```python
from build123d import *

# Parameters (mm, degrees)
SKETCH1_R           = 10.31875
BOSS_EXTRUDE1_DEPTH = 9.525
SKETCH2_R           = 18.2626
BOSS_EXTRUDE2_DEPTH = 19.05
CUT_EXTRUDE1_START  = -2.38125
SKETCH3_OUTSIDE_W   = 50.332
SKETCH3_OUTSIDE_H   = 50.332
SKETCH3_OUTSIDE_R   = 15.1638
CUT_EXTRUDE1_DEPTH  = 14.2875
SKETCH4_R           = 4.7625
CUT_EXTRUDE2_DEPTH  = 14.2875
CIRPATTERN1_COUNT   = 10
CUT_EXTRUDE3_DEPTH  = 39.517213587


with BuildPart() as part:
    # Sketch1 → Boss-Extrude1 (new body)
    with BuildSketch(Plane(origin=(0, 0, 0), x_dir=(0, 0, -1), z_dir=(1, 0, 0))):
        with Locations(Location((0, 0, 0), (0, 0, 180))):
            Circle(SKETCH1_R)
    extrude(amount=BOSS_EXTRUDE1_DEPTH)

    # Sketch2 → Boss-Extrude2 (add)
    with BuildSketch(Plane(origin=(9.525, 0, 0), x_dir=(0, 0, -1), z_dir=(1, 0, 0))):
        with Locations(Location((0, 0, 0), (0, 0, 180))):
            Circle(SKETCH2_R)
    extrude(amount=BOSS_EXTRUDE2_DEPTH)

    # Sketch3 outside → Cut-Extrude1 (cut)
    with BuildSketch(Plane(origin=(28.575, 0, 0), x_dir=(0, 0, -1), z_dir=(1, 0, 0)).offset(CUT_EXTRUDE1_START)):
        Rectangle(SKETCH3_OUTSIDE_W, SKETCH3_OUTSIDE_H)
        Circle(SKETCH3_OUTSIDE_R, mode=Mode.SUBTRACT)
    extrude(amount=-CUT_EXTRUDE1_DEPTH, mode=Mode.SUBTRACT)

    # Sketch4 → Cut-Extrude2 (cut)
    with BuildSketch(Plane.ZY.offset(-26.19375)):
        with Locations((-12.712096792, 8.267008262)):
            Circle(SKETCH4_R)
    cut_extrude2 = extrude(amount=CUT_EXTRUDE2_DEPTH, mode=Mode.SUBTRACT)

    # CirPattern1: Cut-Extrude2 ×10 about axis
    cirpattern1_axis = Axis((0, 0, 0), (1, 0, 0))
    for i in range(1, CIRPATTERN1_COUNT):
        add(cut_extrude2.rotate(cirpattern1_axis, i * 360 / CIRPATTERN1_COUNT), mode=Mode.SUBTRACT)

    # Sketch5 → Cut-Extrude3 (cut, through all)
    with BuildSketch(Plane.ZY):
        Polygon((-7.332348419, 0), (-3.666174209, -6.35), (3.666174209, -6.35), (7.332348419, 0), (3.666174209, 6.35), (-3.666174209, 6.35), align=None)
    extrude(amount=-CUT_EXTRUDE3_DEPTH, mode=Mode.SUBTRACT)


solid = part.part
```
Can you work these out from the model? Positions are in its coordinate system, mm. A direction names the side the tool comes from. Round coordinates to 2 decimals unless told otherwise and drop trailing zeros. Order: outer loops, then holes, each group sorted by start corner. A loop starts at its lowest first (then second) coordinate and runs counter-clockwise, first axis right, second up. Notation, with made-up numbers: (21.5, 70) -> (35.5, 70) arc R9 ccw to (35.5, 74) -> close; hole circle Ø6 at (26, 68.25). An arc over 180 degrees is marked (long way). Return JSON: item names as keys, results as strings. Group by question number.
1. If we section it at B-B, the plane z = 0: Write out the boundary of the cut face in (x, y) (3 decimals), then the cut area to 3 significant figures.
2. I need wall thicknesses on line 1 (X direction, y = 7.5, z = 12) (3 decimals); line 2 (Y direction, x = 2.5, z = 3); line 3 (Y direction, x = 5.5, z = 0). Which ranges of each line are inside material? Lowest first, please. Write a range as [from, to].
3. Which directions (+Z, -Z, +X, -X, +Y, -Y) give clear straight access to the entire face, cutting with the end or side of a thin tool? Please do faces 4 (the face through (14.087, 3.131, 5.525)), 5 (the face through (19.15, -9.688, 3.788)), 6 (the face through (19.15, -0.609, -10.384)), 7 (the face through (11.906, -8, -8)), 8 (the face through (19.15, 9.688, -3.788)).
4. If we section it at D-D, the plane x = 10: Write out the boundary of the cut face in (y, z), then the cut area to 3 significant figures.
5. Will these pins go through, and if not, where does the flat tip stop? pin 1 (1 mm diameter, centred on x = 14, z = 12, fed in from +Y); pin 2 (5 mm diameter, centred on y = 8.5, z = -11.5, fed in from -X) (3 decimals); pin 3 (1 mm diameter, centred on x = 10.5, z = -0.5, fed in from -Y); pin 4 (1 mm diameter, centred on y = -4.5, z = -1, fed in from -X).
6. We'd pull the mould along Z, two halves only. Please class faces 1 (the face through (4.7, -10.23, -1.34)), 2 (the face through (14, 6.35, 0)), 3 (the face through (9.525, 8, 8)): released by +Z, released by -Z, zero draft, split by the parting line, or undercut.
7. If we section it at C-C, the plane y = -2.5: Write out the boundary of the cut face in (x, z) (3 decimals).
Output values:
{
 "1": {"outline": "(0, -10.319) -> (9.525, -10.319) -> (9.525, -18.263) -> (11.906, -18.263) -> (11.906, -11.961) -> (26.194, -11.961) -> (26.194, -18.263) -> (28.575, -18.263) -> (28.575, -6.35) -> (0, -6.35) -> close; (0, 6.35) -> (28.575, 6.35) -> (28.575, 18.263) -> (26.194, 18.263) -> (26.194, 11.961) -> (11.906, 11.961) -> (11.906, 18.263) -> (9.525, 18.263) -> (9.525, 10.319) -> (0, 10.319) -> close", "area": "349 mm²"},
 "2": {"line 1": "[9.525, 11.906], [26.194, 28.575]", "line 2": "[-9.87, -6.35], [6.35, 9.87]", "line 3": "[-10.32, -6.35], [6.35, 10.32]"},
 "3": {"face 4": "+X, -X", "face 5": "-Y", "face 6": "-Z", "face 7": "none", "face 8": "+Y"},
 "4": {"outline": "circle Ø36.53 at (0, 0); hole (-6.35, -3.67) -> (0, -7.33) -> (6.35, -3.67) -> (6.35, 3.67) -> (0, 7.33) -> (-6.35, 3.67) -> close", "area": "908 mm²"},
 "5": {"pin 1": "y = 4.83", "pin 2": "x = 9.525", "pin 3": "y = -18.26", "pin 4": "through"},
 "6": {"face 1": "split by the parting line", "face 2": "undercut", "face 3": "zero draft"},
 "7": {"outline": "(0, -10.011) -> (9.525, -10.011) -> (9.525, -18.091) -> (11.906, -18.091) -> (11.906, -10.701) -> (26.194, -10.701) -> (26.194, -18.091) -> (28.575, -18.091) -> (28.575, -5.889) -> (0, -5.889) -> close; (0, 5.889) -> (28.575, 5.889) -> (28.575, 18.091) -> (26.194, 18.091) -> (26.194, 11.694) -> (11.906, 11.694) -> (11.906, 18.091) -> (9.525, 18.091) -> (9.525, 10.011) -> (0, 10.011) -> close"}
}
